Design review of the part built by this model. Coordinates are the model's own, in mm. A direction names the side the tool comes from. Give positions to 0.01 mm unless a question says otherwise; leave off trailing zeros. Order: outer loops, then holes, each group sorted by start corner. A loop starts at its lowest first (then second) coordinate and runs counter-clockwise, first axis right, second up. Notation, with made-up numbers: (-11.5, 0.25) -> (41.5, 0.25) arc R18 cw to (41.5, 27.25) -> close; hole circle Ø6 at (22, -25.75). An arc over 180 degrees is marked (long way). Use a Markdown table: item, result. Add a question column.
```python
from build123d import *

# Parameters (mm, degrees)
BOSS_EXTRUDE1_DEPTH = 1.65
FILLET1_R           = 0.5


with BuildPart() as part:
    # Sketch1 → Boss-Extrude1 (new, symmetric)
    with BuildSketch(Plane.XY):
        with BuildLine():
            Line((2.1, 0), (2.1, 9.7))
            Line((2.1, 9.7), (-2.1, 9.7))
            Line((-2.1, 9.7), (-2.1, 0))
            ThreePointArc((-2.1, 0), (0, -2.1), (2.1, 0))
        make_face()
        with BuildLine():
            Line((1, 0), (1, 2.2))
            ThreePointArc((1, 2.2), (0, 3.2), (-1, 2.2))
            Line((-1, 2.2), (-1, 0))
            ThreePointArc((-1, 0), (0, -1), (1, 0))
        make_face(mode=Mode.SUBTRACT)
    extrude(amount=BOSS_EXTRUDE1_DEPTH, both=True)

    # Sketch2 → Revolve1 (revolve)
    with BuildSketch(Plane.XY, mode=Mode.PRIVATE) as revolve1_sk:
        Polygon((0, 13.5), (5.69, 13.5), (5.69, 11), (1.62, 11), (1.62, 9.7), (0, 9.7), align=None)
    revolve(revolve1_sk.sketch.rotate(Axis((0, 9.7, 0), (0, 1, 0)), 90), axis=Axis((0, 9.7, 0), (0, 1, 0)))

    # Fillet1
    fillet1_edges = [part.edges().sort_by_distance(p)[0] for p in [
        (2.1, 4.85, 1.65),
        (-2.1, 4.85, 1.65),
        (2.1, 4.85, -1.65),
        (0, -2.1, -1.65),
        (-2.1, 4.85, -1.65),
        (0, -2.1, 1.65),
    ]]
    fillet(fillet1_edges, radius=FILLET1_R)


solid = part.part
```
1) Add section B-B (z = 0). Give the boundary of the cut face in (x, y).
2) The part is to be moulded in two halves that separate along Y. For faces 5 (the flat face through (0.96, 9.7, 1.49)), 6 (the flat face through (0, 13.5, 0)), 7 (the flat face through (2.1, 5, 0)), say which applies: +Y half, -Y half, draft (parallel to the pull), parting line (faces both ways), or undercut.
3) Insertion check: pin 1 (2.5 mm diameter, centred on y = 3, z = -0.5, fed in from +X); pin 2 (3.5 mm diameter, centred on x = 0.5, y = 6, fed in from -Z); pin 3 (3.5 mm diameter, centred on x = 0.5, y = 6.5, fed in from +Z); pin 4 (1.5 mm diameter, centred on y = 0.5, z = -2.5, fed in from -X). Each pin has a flat end and moves straight along its axis. Give the tip position at first contact, or say it passes through.
4) Machinability: for faces 1 (the flat face through (0, 5, -1.65)), 2 (the cylindrical face through (0, 3.2, 0)), 3 (the cylindrical face through (1.58, 10.34, 0.35)), 4 (the flat face through (0, 5, 1.65)), which of the approach directions +Z, -Z, +X, -X, +Y, -Y give a long, thin tool a straight path to every point of the face, cutting with its end or side? Answer none if there is none.
5) Add section D-D (y = 4.75). Give the boundary of the cut face in (x, z), then the cut area to 3 significant figures.
6) Add section A-A (y = 1). Give the boundary of the cut face in (x, z), then the cut area to 3 significant figures.
7) For L1, parallel to Y at x = 4.25, z = 0.25; L2, parallel to X at y = 1.25, z = -1.5; L3, parallel to X at y = 6, z = 1, list the stretches that pass through material, from the lowest coordinate up. Write a range as [from, to].
Worked answers:
| question | item | result |
|---|---|---|
| 1 | outline | (-5.69, 11) -> (-1.62, 11) -> (-1.62, 9.7) -> (-2.1, 9.7) -> (-2.1, 0) arc R2.1 ccw to (2.1, 0) -> (2.1, 9.7) -> (1.62, 9.7) -> (1.62, 11) -> (5.69, 11) -> (5.69, 13.5) -> (-5.69, 13.5) -> close; hole (-1, 0) arc R1 ccw to (1, 0) -> (1, 2.2) arc R1 ccw to (-1, 2.2) -> close |
| 2 | face 5 | undercut |
| 2 | face 6 | +Y half |
| 2 | face 7 | draft |
| 3 | pin 1 | x = 2.1 |
| 3 | pin 2 | z = -1.65 |
| 3 | pin 3 | z = 1.65 |
| 3 | pin 4 | through |
| 4 | face 1 | -Z, +X, -X, -Y |
| 4 | face 2 | +Z, -Z |
| 4 | face 3 | none |
| 4 | face 4 | +Z, +X, -X, -Y |
| 5 | outline | (-2.1, -1.15) arc R0.5 ccw to (-1.6, -1.65) -> (1.6, -1.65) arc R0.5 ccw to (2.1, -1.15) -> (2.1, 1.15) arc R0.5 ccw to (1.6, 1.65) -> (-1.6, 1.65) arc R0.5 ccw to (-2.1, 1.15) -> close |
| 5 | area | 13.6 mm^2 |
| 6 | outline | (-2.1, -1.15) arc R0.5 ccw to (-1.6, -1.65) -> (-1, -1.65) -> (-1, 1.65) -> (-1.6, 1.65) arc R0.5 ccw to (-2.1, 1.15) -> close; (1, -1.65) -> (1.6, -1.65) arc R0.5 ccw to (2.1, -1.15) -> (2.1, 1.15) arc R0.5 ccw to (1.6, 1.65) -> (1, 1.65) -> close |
| 6 | area | 7.05 mm^2 |
| 7 | L1 | [11, 13.5] |
| 7 | L2 | [-1.96, -1], [1, 1.96] |
| 7 | L3 | [-2.1, 2.1] |
